```python
from build123d import *

# Parameters (mm, degrees)
SKETCH_1_W               = 30
SKETCH_1_H               = 15
SKETCH_1_W_2             = 26
SKETCH_1_H_2             = 11
EXTRUDE_1_DEPTH          = 140
SKETCH_2_R               = 2.15
CUT_EXTRUDE_1_DEPTH      = 144.961800489
CUT_EXTRUDE_2_DEPTH      = 144.961800489
CUT_EXTRUDE_2_DEPTH_BACK = 144.961800489
SKETCH_3_R               = 2.15
SKETCH_4_R               = 2.1
CUT_EXTRUDE_3_DEPTH      = 144.961800489
SKETCH_5_R               = 2.1
CUT_EXTRUDE_4_DEPTH      = 144.961800489
SKETCH_6_R               = 2.5
CUT_EXTRUDE_5_DEPTH      = 144.961800489


with BuildPart() as part:
    # 草图1 → 凸台-拉伸1 (new body)
    with BuildSketch(Plane(origin=(0, 0, 0), x_dir=(0, 0, -1), z_dir=(1, 0, 0))):
        with Locations((15, 7.5)):
            Rectangle(SKETCH_1_W, SKETCH_1_H)
        with Locations((15, 7.5)):
            Rectangle(SKETCH_1_W_2, SKETCH_1_H_2, mode=Mode.SUBTRACT)
    extrude(amount=EXTRUDE_1_DEPTH)

    # 草图2 → 切除-拉伸1 (cut, through all)
    with BuildSketch(Plane.XZ):
        with Locations(Location((19.1, -7, 0), (0, 0, 270))):
            Circle(SKETCH_2_R)
        with Locations(Location((19.1, -23, 0), (0, 0, 270))):
            Circle(SKETCH_2_R)
        with Locations(Location((45.3, -23, 0), (0, 0, 270))):
            Circle(SKETCH_2_R)
        with Locations(Location((45.3, -7, 0), (0, 0, 270))):
            Circle(SKETCH_2_R)
    extrude(amount=-CUT_EXTRUDE_1_DEPTH, mode=Mode.SUBTRACT)

    # 草图3 → 切除-拉伸2 (cut, two sides: drawn at the far end of the back side and taken through both)
    with BuildSketch(Plane.XZ.offset(-CUT_EXTRUDE_2_DEPTH_BACK)):
        with Locations(Location((94.7, -7, 0), (0, 0, 270))):
            Circle(SKETCH_3_R)
        with Locations(Location((120.9, -7, 0), (0, 0, 270))):
            Circle(SKETCH_3_R)
        with Locations(Location((120.9, -23, 0), (0, 0, 270))):
            Circle(SKETCH_3_R)
        with Locations(Location((94.7, -23, 0), (0, 0, 270))):
            Circle(SKETCH_3_R)
    extrude(amount=CUT_EXTRUDE_2_DEPTH + CUT_EXTRUDE_2_DEPTH_BACK, mode=Mode.SUBTRACT)

    # 草图4 → 切除-拉伸3 (cut, through all)
    with BuildSketch(Plane.XZ):
        with Locations(Location((131, -9, 0), (0, 0, 270))):
            Circle(SKETCH_4_R)
        with Locations(Location((131, -21, 0), (0, 0, 270))):
            Circle(SKETCH_4_R)
    extrude(amount=-CUT_EXTRUDE_3_DEPTH, mode=Mode.SUBTRACT)

    # 草图5 → 切除-拉伸4 (cut, through all)
    with BuildSketch(Plane.XZ):
        with Locations(Location((9, -9, 0), (0, 0, 270))):
            Circle(SKETCH_5_R)
        with Locations(Location((9, -21, 0), (0, 0, 270))):
            Circle(SKETCH_5_R)
    extrude(amount=-CUT_EXTRUDE_4_DEPTH, mode=Mode.SUBTRACT)

    # 草图6 → 切除-拉伸5 (cut, through all)
    with BuildSketch(Plane.XY):
        with Locations((4.5, 7.4)):
            Circle(SKETCH_6_R)
        with Locations((34.5, 7.4)):
            Circle(SKETCH_6_R)
        with Locations((105.5, 7.4)):
            Circle(SKETCH_6_R)
        with Locations((135.5, 7.4)):
            Circle(SKETCH_6_R)
    extrude(amount=-CUT_EXTRUDE_5_DEPTH, mode=Mode.SUBTRACT)


solid = part.part
```
Can you work these out from the model? Positions are in its coordinate system, mm. A direction names the side the tool comes from. Round coordinates to 2 decimals unless told otherwise and drop trailing zeros. Loops run counter-clockwise (first coordinate to the right, second up) from the corner with the lowest first, then second, coordinate; pieces in that order, holes last.
Item 1: Suppose I cut it at A-A, the plane x = 34.5. Write out the boundary of the cut face in (y, z).
Item 2: Suppose I cut it at B-B, the plane x = 19.1. Write out the boundary of the cut face in (y, z).
Item 3: If we mould it in two halves opening along Z, with no side actions, what happens to faces 1 (the cylindrical face through (137.885, 8.151, -0.986)), 2 (the cylindrical face through (123.03, 1.01, -22.72)), 3 (the flat face through (69, 7, -30))? For each: +Z half, -Z half, draft (parallel to the pull), parting line (faces both ways), or undercut.
Item 4: Suppose I cut it at C-C, the plane x = 65. Write out the boundary of the cut face in (y, z).
Item 5: Which directions (+Z, -Z, +X, -X, +Y, -Y) give clear straight access to the entire face, cutting with the end or side of a thin tool? Please do faces 4 (the cylindrical face through (43.39, 13.99, -7.99)), 5 (the flat face through (69, 2, -15)).
Item 6: Please list where these lines run through material, in increasing order: L1, parallel to Z at x = 94.7, y = 13.5; L2, parallel to Z at x = 131, y = 14.5; L3, parallel to Y at x = 13, z = -26.5.
Reported:
1. outline: (0, -30) - (4.9, -30) - (4.9, -28) - (2, -28) - (2, -2) - (4.9, -2) - (4.9, 0) - (0, 0) - close; (9.9, -30) - (15, -30) - (15, 0) - (9.9, 0) - (9.9, -2) - (13, -2) - (13, -28) - (9.9, -28) - close
2. outline: (0, -30) - (15, -30) - (15, -25.15) - (13, -25.15) - (13, -28) - (2, -28) - (2, -25.15) - (0, -25.15) - close; (0, -20.85) - (2, -20.85) - (2, -9.15) - (0, -9.15) - close; (0, -4.85) - (2, -4.85) - (2, -2) - (13, -2) - (13, -4.85) - (15, -4.85) - (15, 0) - (0, 0) - close; (13, -20.85) - (15, -20.85) - (15, -9.15) - (13, -9.15) - close
3. face 1: draft
3. face 2: undercut
3. face 3: -Z half
4. outline: (0, -30) - (15, -30) - (15, 0) - (0, 0) - close; hole (2, -28) - (13, -28) - (13, -2) - (2, -2) - close
5. face 4: +Y, -Y
5. face 5: +X, -X
6. L1: z = -30 to -25.15, -20.85 to -9.15, -4.85 to 0
6. L2: z = -30 to -23.1, -18.9 to -11.1, -6.9 to 0
6. L3: y = 0 to 2, 13 to 15
